Here's the drawing with two shaded views (mm, measured from the low corner). I have some questions. Coordinates: 2 decimals unless noted, no trailing zeros. Write each loop counter-clockwise with the first axis right and the second up, starting at its lowest first coordinate (ties: lowest second). Pieces come first, ordered by that corner, then holes.
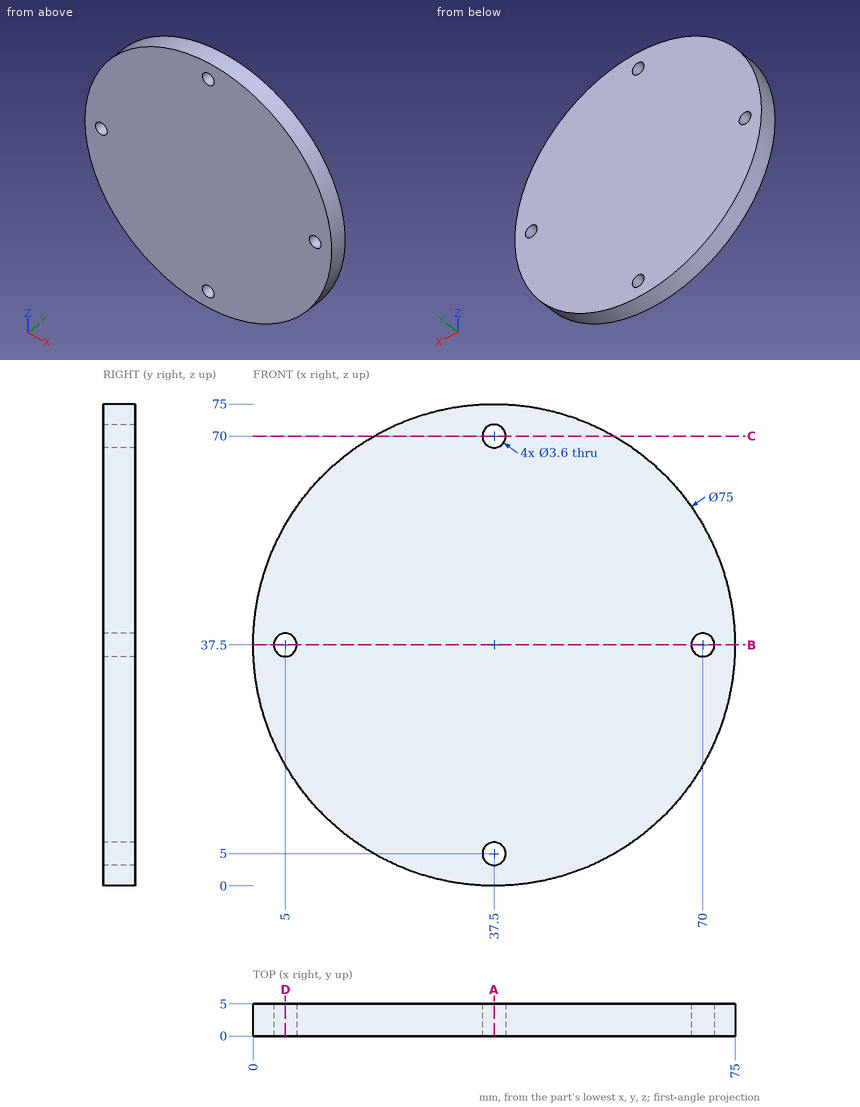
Item 1: If I drill on line 1 along Z through (x, y) = (37.5, 3.9); line 2 along Z through (x, y) = (69, 3.9); line 3 along X through (y, z) = (2.3, 70), over which ranges is the centre line in solid material (lowest first)?
Item 2: I want a section at B-B, the plane z = 37.5. List the corners of the cut face in (x, y) for me.
Item 3: I want a section at D-D, the plane x = 5. List the corners of the cut face in (y, z) for me, then the cut area to 3 significant figures.
Item 4: Will these pins go through, and if not, where does the flat tip stop? pin 1 Ø3 at (x, z) = (37.5, 70) entering from +Y; pin 2 Ø3 at (y, z) = (1.5, 45.5) entering from -X; pin 3 Ø1 at (x, y) = (13.5, 1.5) entering from -Z; pin 4 Ø1.5 at (x, y) = (50.5, 1) entering from -Z.
Item 5: I want a section at A-A, the plane x = 37.5. List the corners of the cut face in (y, z) for me, then the cut area to 3 significant figures.
Item 6: I want a section at C-C, the plane z = 70. List the corners of the cut face in (x, y) for me, then the cut area to 3 significant figures.
Taken from the geometry:
1. line 1: z = 0 to 3.2, 6.8 to 68.2, 71.8 to 75
1. line 2: z = 17.15 to 36, 39 to 57.85
1. line 3: x = 18.79 to 35.7, 39.3 to 56.21
2. outline: (0, 0) - (3.2, 0) - (3.2, 5) - (0, 5) - close; (6.8, 0) - (68.2, 0) - (68.2, 5) - (6.8, 5) - close; (71.8, 0) - (75, 0) - (75, 5) - (71.8, 5) - close
3. outline: (0, 18.79) - (5, 18.79) - (5, 35.7) - (0, 35.7) - close; (0, 39.3) - (5, 39.3) - (5, 56.21) - (0, 56.21) - close
3. area: 169 mm2
4. pin 1: passes through
4. pin 2: stops at x = 0.57
4. pin 3: stops at z = 8.28
4. pin 4: stops at z = 2.06
5. outline: (0, 0) - (5, 0) - (5, 3.2) - (0, 3.2) - close; (0, 6.8) - (5, 6.8) - (5, 68.2) - (0, 68.2) - close; (0, 71.8) - (5, 71.8) - (5, 75) - (0, 75) - close
5. area: 339 mm2
6. outline: (18.79, 0) - (35.7, 0) - (35.7, 5) - (18.79, 5) - close; (39.3, 0) - (56.21, 0) - (56.21, 5) - (39.3, 5) - close
6. area: 169 mm2
